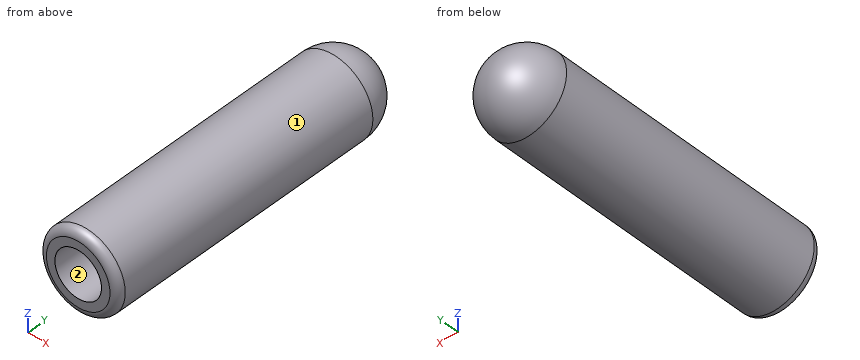
Autodesk Fusion 360 part; units mm, degrees
sketch "Sketch1" plane through (0, 0, 0) normal (0, 1, 0) x (1, 0, 0)
  circle A0 centre (0, 0) radius 2.5
  dimension "d1" = 5
extrude "Extrude1" add sketch "Sketch1" along normal blind 20
sketch "Sketch2" plane through (0, 0, 0) normal (0, 0, 1) x (1, 0, 0)
  line L0 (0, 0) -> (0, 15)
  line L1 (0, 15) -> (0, 17.5)
  dimension "d4" = 15
  dimension "d5" = 2.5
fillet "Fillet1" radius 2.5 1 faces at (-0.8863, 20, -0.2321)
sketch "Sketch3" plane through (0, 0, 0) normal (0, -1, 0) x (1, 0, 0)
  circle A0 centre (0, 0) radius 2.5
  circle A1 centre (0, 0) radius 1.5
  dimension "d8" = 3
hole "Hole1" at (0, 0, 0) direction (0, 1, 0) diameter 2.93 depth 17.5 tip angle 180
fillet "Fillet2" radius 0.5 1 edges at (-2.3308, 0, 0.904)
The listing builds one solid part. Answer for the finished solid, in the listing's coordinates (mm). Face numbers are marked on the shaded views. Coordinates: 2 decimals unless noted, no trailing zeros. Loops run counter-clockwise (first coordinate to the right, second up) from the corner with the lowest first, then second, coordinate; pieces in that order, holes last.
1) A flat-ended cylindrical pin translates along its axis: pin 1 Ø0.9 at (x, z) = (-0.5, -0.5) entering from -Y. Find the tip coordinate at first contact, or state that the pin passes through.
2) Find section C-C on y = 4.25. Write down the section's boundary in (x, z) (3 decimals), then the cut area to 3 significant figures.
3) Find section B-B on z = 0. Write down the section's boundary in (x, y) (3 decimals).
4) Find the intervals of material crossed by L1, parallel to X at y = 7.75, z = 0 (3 decimals); L2, parallel to Z at x = 0.1, y = 15.75; L3, parallel to Z at x = 0.65, y = 5, in increasing order.
5) Find section A-A on x = 0. Write down the section's boundary in (y, z) (3 decimals).
6) Determine the mould class of the marked faces 1 and 2 for opening direction Z: pulls with the +Z half, pulls with the -Z half, needs draft (parallel to the pull), parting line crosses it, or undercut.
Values:
1. pin 1: stops at y = 17.5
2. outline: circle Ø5 at (0, 0); hole circle Ø2.93 at (0, 0)
2. area: 12.9 mm2
3. outline: (-2.5, 0.5) arc R0.5 ccw to (-2, 0) - (-1.465, 0) - (-1.465, 17.5) - (1.465, 17.5) - (1.465, 0) - (2, 0) arc R0.5 ccw to (2.5, 0.5) - (2.5, 17.5) arc R2.5 ccw to (-2.5, 17.5) - close
4. L1: x = -2.5 to -1.465, 1.465 to 2.5
4. L2: z = -2.5 to -1.46, 1.46 to 2.5
4. L3: z = -2.41 to -1.31, 1.31 to 2.41
5. outline: (0, -2) arc R0.5 ccw to (0.5, -2.5) - (17.5, -2.5) arc R2.5 ccw to (17.5, 2.5) - (0.5, 2.5) arc R0.5 ccw to (0, 2) - (0, 1.465) - (17.5, 1.465) - (17.5, -1.465) - (0, -1.465) - close
6. face 1: parting line crosses it
6. face 2: undercut
